Geometry check sheet. Reference: drawing and pictorial views, mm from the part's lowest x, y, z. A direction names the side the tool comes from. Coordinates: 2 decimals unless noted, no trailing zeros. Write each loop counter-clockwise with the first axis right and the second up, starting at its lowest first coordinate (ties: lowest second). Pieces come first, ordered by that corner, then holes. Notation, with made-up numbers: M -36.5,-4.5 L 4.5,-4.5 A26 ccw 4.5,11.5 Z; hole C 77.25,89 d5. An arc over 180 degrees is marked long. One line per item, written item: value.
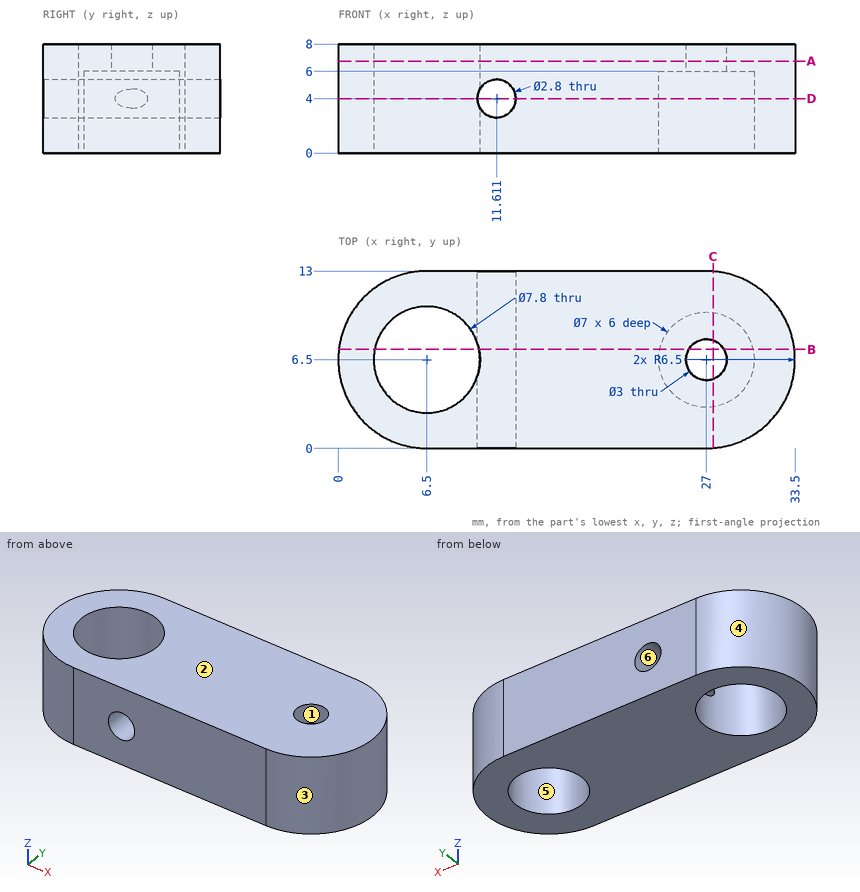
Item 1: Scan lines: line 1 (Y direction, x = 27, z = 4.25); line 2 (Y direction, x = 6.5, z = 3.75); line 3 (X direction, y = 5.5, z = 1). Record each from-to range of solid material in increasing order.
The answers:
line 1: y = 0 to 3, 10 to 13
line 2: y = 0 to 2.6, 10.4 to 13
line 3: x = 0.08 to 2.73, 10.27 to 23.65, 30.35 to 33.42
Item 2: Cross-section at A-A, the plane z = 6.75. Enter the section's corners in (x, y), and give its area (3 significant figures).
The answers:
outline: M 6.5,0 L 27,0 A6.5 ccw 27,13 L 6.5,13 A6.5 ccw Z; hole C 6.5,6.5 d7.8; hole C 27,6.5 d3
area: 344 mm²
Item 3: Access from +Z, -Z, +X, -X, +Y, -Y to the whole of each face (thin tool, end or side, straight path). Record for the marked faces 5 and 6.
The answers:
face 5: -Z
face 6: +Y, -Y
Item 4: Cross-section at D-D, the plane z = 4. Enter the section's corners in (x, y), and give its area (3 significant figures).
The answers:
outline: M 6.5,0 L 10.21,0 L 10.21,5.3 A3.9 cw long 10.21,7.7 L 10.21,13 L 6.5,13 A6.5 ccw Z; M 13.01,0 L 27,0 A6.5 ccw 27,13 L 13.01,13 Z; hole C 27,6.5 d7
area: 277 mm²
Item 5: Go/stop test with flat-tipped pins: P1, Ø2, axis at x = 27.5, y = 5, coming from the -Z side; P2, Ø2, axis at y = 9.5, z = 7, coming from the +X side (1 decimal); P3, Ø1, axis at y = 11, z = 7, coming from the +X side. Record where each tip stops, or that it passes through.
The answers:
P1: stops at z = 6
P2: stops at x = 33.2
P3: stops at x = 32.12
Item 6: Draft check along X on the marked faces 1, 2, 3 and 4. Enter one of: released by +X, released by -X, zero draft, split by the parting line, or undercut.
The answers:
face 1: undercut
face 2: zero draft
face 3: released by +X
face 4: released by -X
Item 7: Cross-section at C-C, the plane x = 27.5. Enter the section's corners in (y, z).
The answers:
outline: M 0.02,0 L 3.04,0 L 3.04,6 L 5.09,6 L 5.09,8 L 0.02,8 Z; M 7.91,6 L 9.96,6 L 9.96,0 L 12.98,0 L 12.98,8 L 7.91,8 Z
Item 8: Cross-section at B-B, the plane y = 7.25. Enter the section's corners in (x, z), and give its area (3 significant figures).
The answers:
outline: M 0.04,0 L 2.67,0 L 2.67,8 L 0.04,8 Z; M 10.33,0 L 23.58,0 L 23.58,6 L 25.7,6 L 25.7,8 L 10.33,8 L 10.33,4.56 A1.4 cw long 10.33,3.44 Z; M 28.3,6 L 30.42,6 L 30.42,0 L 33.46,0 L 33.46,8 L 28.3,8 Z
area: 154 mm²
